```python
from build123d import *

# Parameters (mm, degrees)
BASEPLATE_OUTLINE_R = 2.1
BASEPLATE_DEPTH     = 2.8
CUT_EXTRUDE1_REACH  = 115.438
FILLET1_R           = 1
CUT_EXTRUDE2_REACH  = 115.438
SKETCH4_W           = 1.3
SKETCH4_H           = 11.5
SKETCH4_H_2         = 13
BOSS_EXTRUDE1_START = -2.8
BOSS_EXTRUDE1_DEPTH = 2.8


# Read off the part's stored shape, not the designer's step: BasePlate
with BuildPart() as part:
    # BasePlate outline → BasePlate (new body)
    with BuildSketch(Plane(origin=(0, 0, 0), x_dir=(1, 0, 0), z_dir=(0, 1, 0))):
        with BuildLine():
            Line((43.502626614, -5.852332608), (48.792614178, -5.852332608))
            ThreePointArc((48.792614178, -5.852332608), (49.082078508, -5.760021707), (49.264659986, -5.517174213))
            Line((49.264659986, -5.517174213), (50.078201202, -3.187491002))
            ThreePointArc((50.078201202, -3.187491002), (50.26078268, -2.944643509), (50.55024701, -2.852332608))
            Line((50.55024701, -2.852332608), (58.116695703, -2.852332608))
            ThreePointArc((58.116695703, -2.852332608), (58.484685739, -3.013831008), (58.614956567, -3.393999275))
            ThreePointArc((58.614956567, -3.393999275), (64.799237397, -7.61016844), (65.229166667, -0.137781095))
            ThreePointArc((65.229166667, -0.137781095), (65.061014427, 0.043158816), (65, 0.282515593))
            Line((65, 0.282515593), (65, 83.012819192))
            ThreePointArc((65, 83.012819192), (65.061014427, 83.252175969), (65.229166667, 83.433115879))
            ThreePointArc((65.229166667, 83.433115879), (65.940559159, 90.088226551), (59.285448487, 89.376834059))
            ThreePointArc((59.285448487, 89.376834059), (59.104508577, 89.208681819), (58.8651518, 89.147667392))
            Line((58.8651518, 89.147667392), (6.1348482, 89.147667392))
            ThreePointArc((6.1348482, 89.147667392), (5.895491423, 89.208681819), (5.714551513, 89.376834059))
            ThreePointArc((5.714551513, 89.376834059), (-0.940559159, 90.088226551), (-0.229166667, 83.433115879))
            ThreePointArc((-0.229166667, 83.433115879), (-0.061014427, 83.252175969), (0, 83.012819192))
            Line((0, 83.012819192), (0, 0.282515593))
            ThreePointArc((0, 0.282515593), (-0.061014427, 0.043158816), (-0.229166667, -0.137781095))
            ThreePointArc((-0.229166667, -0.137781095), (0.200762603, -7.61016844), (6.385043433, -3.393999275))
            ThreePointArc((6.385043433, -3.393999275), (6.515314261, -3.013831008), (6.883304297, -2.852332608))
            Line((6.883304297, -2.852332608), (14.44975299, -2.852332608))
            ThreePointArc((14.44975299, -2.852332608), (14.73921732, -2.944643509), (14.921798798, -3.187491002))
            Line((14.921798798, -3.187491002), (15.735340014, -5.517174213))
            ThreePointArc((15.735340014, -5.517174213), (15.917921492, -5.760021707), (16.207385822, -5.852332608))
            Line((16.207385822, -5.852332608), (21.497373386, -5.852332608))
            ThreePointArc((21.497373386, -5.852332608), (21.786837716, -5.760021707), (21.969419194, -5.517174213))
            Line((21.969419194, -5.517174213), (22.78296041, -3.187491002))
            ThreePointArc((22.78296041, -3.187491002), (22.965541888, -2.944643509), (23.255006218, -2.852332608))
            Line((23.255006218, -2.852332608), (41.744993782, -2.852332608))
            ThreePointArc((41.744993782, -2.852332608), (42.034458112, -2.944643509), (42.21703959, -3.187491002))
            Line((42.21703959, -3.187491002), (43.030580806, -5.517174213))
            ThreePointArc((43.030580806, -5.517174213), (43.213162284, -5.760021707), (43.502626614, -5.852332608))
        make_face()
        with Locations((2.1, -3.752332608)):
            Circle(BASEPLATE_OUTLINE_R, mode=Mode.SUBTRACT)
        with Locations((62.9, -3.752332608)):
            Circle(BASEPLATE_OUTLINE_R, mode=Mode.SUBTRACT)
        with Locations((2.1, 87.047667392)):
            Circle(BASEPLATE_OUTLINE_R, mode=Mode.SUBTRACT)
        with Locations((62.9, 87.047667392)):
            Circle(BASEPLATE_OUTLINE_R, mode=Mode.SUBTRACT)
    extrude(amount=BASEPLATE_DEPTH)

    # Sketch3 → Cut-Extrude1 (cut, up to next)
    with BuildSketch(Plane(origin=(0, 2.8, 0), x_dir=(1, 0, 0), z_dir=(0, 1, 0)), mode=Mode.PRIVATE) as cut_extrude1_sk1:
        Polygon((4.9, 85.647667392), (4.9, -0.852332608), (22.9, -0.852332608), (22.9, -3.00023804), (42.1, -3.00023804), (42.1, -0.852332608), (62, -0.852332608), (62, 85.647667392), align=None)
    cut_extrude1_tool1 = extrude(cut_extrude1_sk1.sketch, amount=-CUT_EXTRUDE1_REACH, mode=Mode.PRIVATE) & part.part
    add(cut_extrude1_tool1.solids().sort_by_distance((33.442134, 2.8, -42.030646))[0], mode=Mode.SUBTRACT)

    # Fillet1
    fillet1_edges = [part.edges().sort_by_distance(p)[0] for p in [
        (4.9, 1.4, -85.647667392),
        (62, 1.4, 0.852332608),
        (4.9, 1.4, 0.852332608),
    ]]
    fillet(fillet1_edges, radius=FILLET1_R)

    # Sketch4 → Cut-Extrude2 (cut, up to next)
    with BuildSketch(Plane(origin=(0, 2.8, 0), x_dir=(1, 0, 0), z_dir=(0, 1, 0)), mode=Mode.PRIVATE) as cut_extrude2_sk1:
        with Locations((64.35, 54.297667392)):
            Rectangle(SKETCH4_W, SKETCH4_H)
    cut_extrude2_tool1 = extrude(cut_extrude2_sk1.sketch, amount=-CUT_EXTRUDE2_REACH, mode=Mode.PRIVATE) & part.part
    # Sketch4 → Cut-Extrude2 (cut, up to next)
    with BuildSketch(Plane(origin=(0, 2.8, 0), x_dir=(1, 0, 0), z_dir=(0, 1, 0)), mode=Mode.PRIVATE) as cut_extrude2_sk2:
        with Locations((64.35, 10.647667392)):
            Rectangle(SKETCH4_W, SKETCH4_H_2)
    cut_extrude2_tool2 = extrude(cut_extrude2_sk2.sketch, amount=-CUT_EXTRUDE2_REACH, mode=Mode.PRIVATE) & part.part
    add(cut_extrude2_tool1.solids().sort_by_distance((64.35, 2.8, -54.297667))[0], mode=Mode.SUBTRACT)
    add(cut_extrude2_tool2.solids().sort_by_distance((64.35, 2.8, -10.647667))[0], mode=Mode.SUBTRACT)

    # Sketch5 → Boss-Extrude1 (add)
    with BuildSketch(Plane(origin=(0, 2.8, 0), x_dir=(1, 0, 0), z_dir=(0, 1, 0)).offset(BOSS_EXTRUDE1_START)):
        with BuildLine():
            Line((61.334752416, 85.647667392), (60.536822695, 85.647667392))
            ThreePointArc((60.536822695, 85.647667392), (61.162428481, 84.920356368), (62, 84.45255526))
            Line((62, 84.45255526), (62, 85.150300796))
            ThreePointArc((62, 85.150300796), (61.64254034, 85.365765134), (61.334752416, 85.647667392))
        make_face()
    extrude(amount=BOSS_EXTRUDE1_DEPTH)


solid = part.part
```
Here's how the part is built. I have some questions about the finished solid (model axes, mm). A direction names the side the tool comes from. Coordinates: 2 decimals unless noted, no trailing zeros. Order: outer loops, then holes, each group sorted by start corner. A loop starts at its lowest first (then second) coordinate and runs counter-clockwise, first axis right, second up. Notation, with made-up numbers: (12, 74) - (70, 74) arc R30 cw to (70, 112) - close; hole circle Ø4 at (-3, 87). An arc over 180 degrees is marked (long way). One line per question, with ' | ' between items. Start each with the question number.
1. I'm going to push flat-ended pins straight in: pin 1 Ø1 at (y, z) = (2, -32) entering from -X; pin 2 Ø4 at (x, z) = (62.9, 3.75) entering from +Y; pin 3 Ø1 at (y, z) = (1, -18) entering from +X; pin 4 Ø1.4 at (x, y) = (15.5, 1.5) entering from -Z. Where does each tip first touch, or does it pass through?
2. If we section it at A-A (z = -46): Write out the boundary of the cut face in (x, y), and give its area (3 significant figures).
3. If we section it at C-C (x = 2.1): Write out the boundary of the cut face in (y, z), and give its area (3 significant figures).
4. If we mould it in two halves opening along Z, with no side actions, what happens to faces 1 (the flat face through (11, 1, 2.852)), 2 (the flat face through (34, 1, -85.648)), 3 (the flat face through (42.1, 1, 2))? For each: released by +Z, released by -Z, zero draft, split by the parting line, or undercut.
5. Please list where these lines run through material, in increasing order: line 1 along Z through (x, y) = (2.1, 1.9); line 2 along X through (y, z) = (2.4, -4.5); line 3 along X through (y, z) = (0.9, -2.5). Write a range as [from, to].
6. If we section it at D-D (y = 0.6): Give the number of separate pieces and of enclosed holes in the cut face, and give its area (3 significant figures).
7. If we section it at B-B (x = 53): Write out the boundary of the cut face in (y, z).
8. Which directions (+Z, -Z, +X, -X, +Y, -Y) give clear straight access to the entire face, cutting with the end or side of a thin tool? Please do faces 4 (the flat face through (0, 1, -42)), 5 (the flat face through (19, 1, 5.852)), 6 (the flat face through (14, 1, 0.852)), 7 (the flat face through (65, 1, -71)).
Model answer:
1) pin 1: stops at x = 0 | pin 2: passes through | pin 3: stops at x = 65 | pin 4: stops at z = -89.15
2) outline: (0, 0) - (4.9, 0) - (4.9, 2.8) - (0, 2.8) - close; (62, 0) - (65, 0) - (65, 2.8) - (62, 2.8) - close | area: 22.1 mm²
3) outline: (0, -91.35) - (2.8, -91.35) - (2.8, -89.15) - (0, -89.15) - close; (0, -84.95) - (2.8, -84.95) - (2.8, 1.65) - (0, 1.65) - close; (0, 5.85) - (2.8, 5.85) - (2.8, 8.05) - (0, 8.05) - close | area: 255 mm²
4) face 1: released by +Z | face 2: undercut | face 3: zero draft
5) line 1: z = [-91.35, -89.15], [-84.95, 1.65], [5.85, 8.05] | line 2: x = [0, 4.9], [62, 63.7] | line 3: x = [0, 4.9], [62, 65]
6) separate pieces: 1 | enclosed holes: 4 | area: 1,080 mm²
7) outline: (0, -89.15) - (2.8, -89.15) - (2.8, -85.65) - (0, -85.65) - close; (0, 0.85) - (2.8, 0.85) - (2.8, 2.85) - (0, 2.85) - close
8) face 4: -X, +Y, -Y | face 5: +Z, +Y, -Y | face 6: +Y, -Y | face 7: +X, +Y, -Y
